Could you check a few things on this model? Use its own coordinates, in mm. Face numbers are marked on the shaded views. A direction names the side the tool comes from. Coordinates: 2 decimals unless noted, no trailing zeros. Loops run counter-clockwise (first coordinate to the right, second up) from the corner with the lowest first, then second, coordinate; pieces in that order, holes last.
1) Thinking about a two-plate mould opening in Z: for the marked faces 1, 2, 3 and 4, which applies, released by +Z, released by -Z, zero draft, split by the parting line, or undercut?
2) If I drill on line 1 along Z through (x, y) = (58, 9.25); line 2 along X through (y, z) = (6, 2.5); line 3 along X through (y, z) = (1.25, 5), over which ranges is the centre line in solid material (lowest first)?
3) Imagine slicing it at A-A on z = 6. Please give me the cut outline in (x, y).
4) Will these pins go through, and if not, where does the flat tip stop? P1, Ø4, axis at x = 29, y = 9.5, coming from the +Z side; P2, Ø3, axis at x = 13, y = 5, coming from the -Z side; P3, Ø3.5, axis at x = 44, y = 6.5, coming from the -Z side; P4, Ø6, axis at x = 21.5, z = 6, coming from the -Y side.
5) For the marked faces 5, 6 and 7, which set-ups out of +Z, -Z, +X, -X, +Y, -Y let a thin tool reach every point of the face, with its end or its side?
6) Imagine slicing it at C-C on x = 25. Please give me the cut outline in (y, z).
7) Imagine slicing it at D-D on x = 57. Please give me the cut outline in (y, z), plus the area to 3 significant figures.
8) Imagine slicing it at B-B on y = 6.75. Please give me the cut outline in (x, z).
```python
from build123d import *

# Parameters (mm, degrees)
BOSS_EXTRUDE2_DEPTH = 10.5
BOSS_EXTRUDE3_DEPTH = 10.5
FILLET1_R           = 100


with BuildPart() as part:
    # Sketch1 → Boss-Extrude2 (new body)
    with BuildSketch(Plane(origin=(0, 0, 0), x_dir=(1, 0, 0), z_dir=(0, 1, 0))):
        with BuildLine():
            Line((3.5, 3.507264218), (3.5, -3.507264218))
            ThreePointArc((3.5, -3.507264218), (6.023664299, -5.996968064), (9.45, -6.906764966))
            ThreePointArc((9.45, -6.906764966), (13.341155227, -5.869242314), (17.152471347, -7.169785158))
            ThreePointArc((17.152471347, -7.169785158), (17.367404774, -7.330790599), (17.575940883, -7.5))
            Line((17.575940883, -7.5), (18.236470068, -7.5))
            Line((18.236470068, -7.5), (29.643235034, 3.906764966))
            ThreePointArc((29.643235034, 3.906764966), (37.704252339, 4.154252339), (37.456764966, -3.906764966))
            Line((37.456764966, -3.906764966), (25.736470068, -15.627059864))
            Line((25.736470068, -15.627059864), (27.222899263, -17.113489059))
            Line((27.222899263, -17.113489059), (32.492349737, -11.844038585))
            ThreePointArc((32.492349737, -11.844038585), (38.950911947, -8.178365919), (46.267551404, -6.906764966))
            Line((46.267551404, -6.906764966), (57.65, -6.906764966))
            ThreePointArc((57.65, -6.906764966), (61.076335701, -5.996968064), (63.6, -3.507264218))
            Line((63.6, -3.507264218), (63.6, 3.507264218))
            ThreePointArc((63.6, 3.507264218), (61.076335701, 5.996968064), (57.65, 6.906764966))
            Line((57.65, 6.906764966), (55.770931212, 6.906764966))
            ThreePointArc((55.770931212, 6.906764966), (50.476561055, 7.055190286), (45.19882198, 7.5))
            Line((45.19882198, 7.5), (41.924547238, 7.5))
            Line((41.924547238, 7.5), (41.422065041, 8.002482197))
            ThreePointArc((41.422065041, 8.002482197), (38.474068809, 8.503220626), (35.543391077, 9.09697881))
            ThreePointArc((35.543391077, 9.09697881), (33.55, 9.312820811), (31.556608923, 9.09697881))
            ThreePointArc((31.556608923, 9.09697881), (21.501954522, 7.455914007), (11.329068788, 6.906764966))
            Line((11.329068788, 6.906764966), (9.45, 6.906764966))
            ThreePointArc((9.45, 6.906764966), (6.023664299, 5.996968064), (3.5, 3.507264218))
        make_face()
    extrude(amount=BOSS_EXTRUDE2_DEPTH)

    # Sketch4 → Boss-Extrude3 (add)
    with BuildSketch(Plane.XZ):
        with BuildLine():
            ThreePointArc((17.575940883, 7.5), (17.752085177, 7.65383798), (17.922940136, 7.813529932))
            Line((17.922940136, 7.813529932), (16.508443005, 9.228027063))
            ThreePointArc((16.508443005, 9.228027063), (13.612622768, 7.891439794), (10.504365982, 8.606268534))
            Line((10.504365982, 8.606268534), (9.45, 6.906764966))
            ThreePointArc((9.45, 6.906764966), (13.609320969, 5.883604236), (17.575940883, 7.5))
        make_face()
        with BuildLine():
            Line((17.575940883, 7.5), (18.236470068, 7.5))
            Line((18.236470068, 7.5), (17.922940136, 7.813529932))
            ThreePointArc((17.922940136, 7.813529932), (17.752085177, 7.65383798), (17.575940883, 7.5))
        make_face()
        Polygon((21.720364105, 19.643165827), (25.736470068, 15.627059864), (26.69888256, 16.589472356), (27.222899263, 17.113489059), (23.2067933, 21.129595022), align=None)
    extrude(amount=-BOSS_EXTRUDE3_DEPTH)

    # Fillet1
    # the kernel refuses this fillet: 100 mm, written as the material it takes off along each edge
    with BuildSketch(Plane(origin=(10.504365982, -9.09791834, 8.606268534), x_dir=(0.9842985265929657, 0, -0.17651178585838628), z_dir=(0, 1, 0))) as fillet1_piece_1:
        with BuildLine():
            CenterArc((40.530590954, 92.946344003), FILLET1_R, 245.626436409, 2.724892596)
            Line((-0.737828472, 1.85892688), (-1.563196861, 0.037178538))
            ThreePointArc((-1.563196861, 0.037178538), (-2.227841116, 0.191634968), (-1.85892688, -0.737828472))
            Line((-1.85892688, -0.737828472), (0.737828472, -1.85892688))
            ThreePointArc((0.737828472, -1.85892688), (1.819583668, -1.652094823), (2.901338864, -1.85892688))
            Line((2.901338864, -1.85892688), (3.639167336, 0))
        make_face()
    extrude(amount=28.69583668, mode=Mode.SUBTRACT)


solid = part.part
```
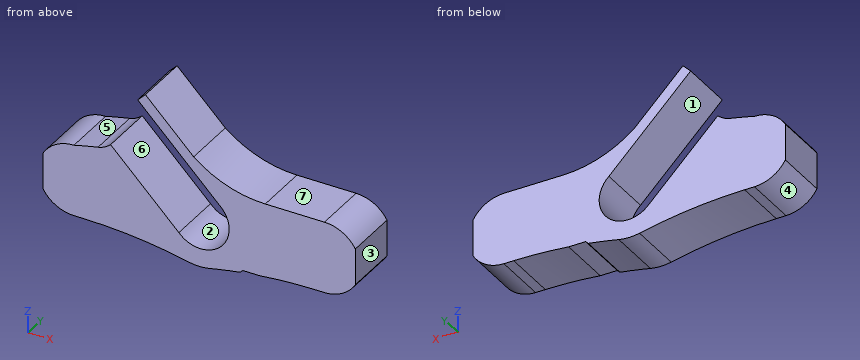
Filled in:
1. face 1: undercut
1. face 2: undercut
1. face 3: zero draft
1. face 4: released by -Z
2. line 1: z = -6.9 to 6.9
2. line 2: x = 3.5 to 23.24, 38.6 to 63.6
2. line 3: x = 4.69 to 20.74, 36.36 to 62.41
3. outline: (6.03, 0) - (19.74, 0) - (19.74, 10.5) - (6.03, 10.5) - close; (35.36, 0) - (61.07, 0) - (61.07, 10.5) - (35.36, 10.5) - close
4. P1: stops at z = 17.34
4. P2: stops at z = -6.96
4. P3: stops at z = -7.5
4. P4: stops at y = 0
5. face 5: +Z, -X, +Y, -Y
5. face 6: +Y, -Y
5. face 7: +Z, +X, +Y, -Y
6. outline: (0, -7.9) - (10.5, -7.9) - (10.5, 0.74) - (0, 0.74) - close; (0, 16.36) - (10.5, 16.36) - (10.5, 19.34) - (0, 19.34) - close
7. outline: (0, -6.91) - (10.5, -6.91) - (10.5, 6.91) - (0, 6.91) - close
7. area: 145 mm2
8. outline: (3.5, -3.51) arc R6.91 ccw to (9.45, -6.91) - (11.33, -6.91) arc R94.5 cw to (31.56, -9.1) arc R9.31 ccw to (35.54, -9.1) arc R94.5 cw to (41.42, -8) - (41.92, -7.5) - (45.2, -7.5) arc R94.5 cw to (55.77, -6.91) - (57.65, -6.91) arc R6.91 ccw to (63.6, -3.51) - (63.6, 3.51) arc R6.91 ccw to (57.65, 6.91) - (46.27, 6.91) arc R21.69 cw to (32.49, 11.84) - (23.21, 21.13) - (21.72, 19.64) - (37.46, 3.91) arc R5.54 cw (long way) to (29.64, -3.91) - (16.51, 9.23) arc R4.93 cw to (14.09, 7.96) arc R100 ccw to (9.45, 6.91) arc R6.91 ccw to (3.5, 3.51) - close
